```python
from build123d import *

# Parameters (mm, degrees)
F2_R     = 9.525
F3_DEPTH = 44.451


with BuildPart() as f1:
    # F0 (on Front) → F1 (revolve)
    with BuildSketch(Plane.XZ):
        Polygon((-63.5, 0), (-46.0375, 0), (-46.0375, 44.45), (-53.975, 44.45), (-53.975, 38.1), (-95.25, 38.1), (-95.25, 1.5875), (-63.5, 1.5875), align=None)
    revolve(axis=Axis((0, 0, 22.225), (0, 0, 1)))

    # F2 (on Top) → F3 (cut, through all)
    with BuildSketch(Plane.XY):
        with Locations((76.2, 0)):
            Circle(F2_R)
        with Locations((0, 76.2)):
            Circle(F2_R)
        with Locations((-76.2, 0)):
            Circle(F2_R)
        with Locations((0, -76.2)):
            Circle(F2_R)
    extrude(amount=F3_DEPTH, mode=Mode.SUBTRACT)


solid = f1.part
```
Build history of the part. All positions in model axes, mm. A direction names the side the tool comes from. Round coordinates to 2 decimals unless told otherwise and drop trailing zeros.
1) Drill centre lines: probe 1 along Y at (x, z) = (3.5, 33); probe 2 along X at (y, z) = (-2, 36); probe 3 along Z at (x, y) = (-63, -63.5). Where is each one in solid material? Low to high.
2) Mould opens along Y. For faces 1 (the cylindrical face through (75.587, 57.958, 19.588)), 2 (the cylindrical face through (4.4, -84.65, 19.59)), 3 (the flat face through (1, -65, 1.587)) say: +Y half, -Y half, draft (parallel to the pull), parting line (faces both ways), or undercut.
3) Band-saw the part on A-A, the plane x = 0. Give the number of separate pieces and of enclosed holes in the cut face, and give its area (3 significant figures).
4) 3-axis set-ups, long thin cutter, end or side, ignore diameter. For faces 4 (the cylindrical face through (39.78, -36.48, 41.23)), 5 (the cylindrical face through (13.77, 61.99, 0.78)), 6 (the flat face through (-33, -33, 0)): which of +Z, -Z, +X, -X, +Y, -Y reach the whole face in a straight line?
5) Pin check, flat tips, straight feed: pin 1 (5 mm diameter, centred on x = 73.5, z = 27, fed in from -Y); pin 2 (6 mm diameter, centred on y = 63.5, z = 9, fed in from +X); pin 3 (25 mm diameter, centred on x = 0, y = -76.2, fed in from -Z). Stop position of each tip, or through.
Ans:
1. probe 1: y = -95.19 to -85.06, -67.34 to -45.9, 45.9 to 67.34, 85.06 to 95.19
1. probe 2: x = -95.23 to -85.51, -66.89 to -45.99, 45.99 to 66.89, 85.51 to 95.23
1. probe 3: z = 1.59 to 38.1
2. face 1: parting line
2. face 2: undercut
2. face 3: draft
3. separate pieces: 4
3. enclosed holes: 0
3. area: 2,360 mm2
4. face 4: +Z
4. face 5: -Z
4. face 6: -Z, +X, -X, +Y, -Y
5. pin 1: stops at y = -63.49
5. pin 2: stops at x = 73.57
5. pin 3: stops at z = 1.59
